Verification items for the finished model (mm, model axes). Give positions to 0.01 mm unless a question says otherwise; leave off trailing zeros. Write each loop counter-clockwise with the first axis right and the second up, starting at its lowest first coordinate (ties: lowest second). Pieces come first, ordered by that corner, then holes. Notation, with made-up numbers: (87.5, 3.5) -> (116.5, 3.5) arc R33 ccw to (116.5, 38.5) -> close; hole circle Ø9 at (54, 65). An arc over 180 degrees is marked (long way). Answer as CSV lines item,"result".
```python
from build123d import *

# Parameters (mm, degrees)
SKETCH_1_W          = 9
SKETCH_1_H          = 6.5
EXTRUDE_1_DEPTH     = 120
SKETCH_2_R          = 1.5
CUT_EXTRUDE_1_DEPTH = 100


with BuildPart() as part:
    # 草图1 → 凸台-拉伸1 (new body)
    with BuildSketch(Plane.XY):
        with Locations((4.5, 3.25)):
            Rectangle(SKETCH_1_W, SKETCH_1_H)
    extrude(amount=EXTRUDE_1_DEPTH)

    # 草图2 → 切除-拉伸1 (cut)
    with BuildSketch(Plane(origin=(0, 6.5, 0), x_dir=(1, 0, 0), z_dir=(0, 1, 0))):
        with Locations(Location((4.5, -115, 0), (0, 0, 270))):
            Circle(SKETCH_2_R)
        with Locations(Location((4.5, -95, 0), (0, 0, 270))):
            Circle(SKETCH_2_R)
        with Locations(Location((4.5, -75, 0), (0, 0, 270))):
            Circle(SKETCH_2_R)
        with Locations(Location((4.5, -55, 0), (0, 0, 270))):
            Circle(SKETCH_2_R)
        with Locations(Location((4.5, -35, 0), (0, 0, 270))):
            Circle(SKETCH_2_R)
        with Locations(Location((4.5, -15, 0), (0, 0, 270))):
            Circle(SKETCH_2_R)
    extrude(amount=-CUT_EXTRUDE_1_DEPTH, mode=Mode.SUBTRACT)


solid = part.part
```
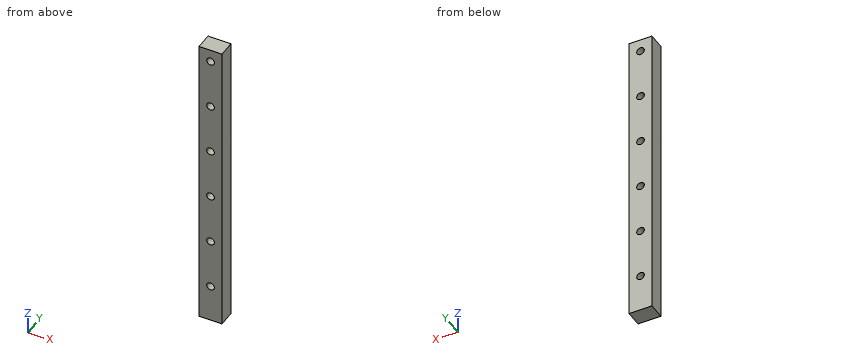
1) Scan lines: line 1 along X through (y, z) = (3, 35); line 2 along X through (y, z) = (2, 114.5). Record each from-to range of solid material in increasing order.
Reported:
line 1,"0 to 3, 6 to 9"
line 2,"0 to 3.09, 5.91 to 9"
2) Section check B-B (y = 2.75). Record the boundary of the cut face in (x, z), and give its area (3 significant figures).
Reported:
outline,"(0, 0) -> (9, 0) -> (9, 120) -> (0, 120) -> close; hole circle Ø3 at (4.5, 15); hole circle Ø3 at (4.5, 35); hole circle Ø3 at (4.5, 55); hole circle Ø3 at (4.5, 75); hole circle Ø3 at (4.5, 95); hole circle Ø3 at (4.5, 115)"
area,"1,040 mm²"
3) Section check C-C (z = 55.5). Record the boundary of the cut face in (x, y), and give its area (3 significant figures).
Reported:
outline,"(0, 0) -> (3.09, 0) -> (3.09, 6.5) -> (0, 6.5) -> close; (5.91, 0) -> (9, 0) -> (9, 6.5) -> (5.91, 6.5) -> close"
area,"40.1 mm²"
4) Section check A-A (z = 95). Record the boundary of the cut face in (x, y).
Reported:
outline,"(0, 0) -> (3, 0) -> (3, 6.5) -> (0, 6.5) -> close; (6, 0) -> (9, 0) -> (9, 6.5) -> (6, 6.5) -> close"
